Read the model definition and answer for the solid it produces. Units are mm, in the model's axes. A direction names the side the tool comes from. Give positions to 0.01 mm unless a question says otherwise; leave off trailing zeros. Order: outer loops, then holes, each group sorted by start corner. A loop starts at its lowest first (then second) coordinate and runs counter-clockwise, first axis right, second up. Notation, with made-up numbers: (-33, 27.5) - (-29, 27.5) arc R11 cw to (-29, 48.5) - close; hole circle Ø3 at (79.25, -7.5). An arc over 180 degrees is marked (long way). Write item = value, one per line.
```python
from build123d import *

# Parameters (mm, degrees)
SKETCH1_W           = 50
SKETCH1_H           = 50
BOSS_EXTRUDE1_DEPTH = 2
SKETCH2_W           = 50
SKETCH2_H           = 50
SKETCH2_W_2         = 38
SKETCH2_H_2         = 38
BOSS_EXTRUDE2_DEPTH = 23


with BuildPart() as part:
    # Sketch1 → Boss-Extrude1 (new body)
    with BuildSketch(Plane.XY):
        Rectangle(SKETCH1_W, SKETCH1_H)
        with BuildLine():
            Line((12.263455967, 16.763455967), (-12.263455967, 16.763455967))
            ThreePointArc((-12.263455967, 16.763455967), (-15.445436483, 15.445436483), (-16.763455967, 12.263455967))
            Line((-16.763455967, 12.263455967), (-16.763455967, -12.263455967))
            ThreePointArc((-16.763455967, -12.263455967), (-15.445436483, -15.445436483), (-12.263455967, -16.763455967))
            Line((-12.263455967, -16.763455967), (12.263455967, -16.763455967))
            ThreePointArc((12.263455967, -16.763455967), (15.445436483, -15.445436483), (16.763455967, -12.263455967))
            Line((16.763455967, -12.263455967), (16.763455967, 12.263455967))
            ThreePointArc((16.763455967, 12.263455967), (15.445436483, 15.445436483), (12.263455967, 16.763455967))
        make_face(mode=Mode.SUBTRACT)
    extrude(amount=-BOSS_EXTRUDE1_DEPTH)

    # Sketch2 → Boss-Extrude2 (add)
    with BuildSketch(Plane(origin=(0, 0, -2), x_dir=(-1, 0, 0), z_dir=(0, 0, -1))):
        Rectangle(SKETCH2_W, SKETCH2_H)
        Rectangle(SKETCH2_W_2, SKETCH2_H_2, mode=Mode.SUBTRACT)
    extrude(amount=BOSS_EXTRUDE2_DEPTH)


solid = part.part
```
1. Section D-D (y = -18) is taken. Determine the outline of the cut face in (x, z), and give its area (3 significant figures).
Recorded:
outline = (-25, -25) - (-19, -25) - (-19, -2) - (19, -2) - (19, -25) - (25, -25) - (25, 0) - (-25, 0) - close
area = 376 mm^2
2. Straight lines are drawn through the part: L1, parallel to Y at x = 12.5, z = -10.5; L2, parallel to Z at x = 18.5, y = -4. For each, find the intervals that lie inside material, in ascending order. Write a range as [from, to].
Recorded:
L1 = [-25, -19], [19, 25]
L2 = [-2, 0]
3. Flat-ended cylindrical pins translate along their axes: pin 1 (6 mm diameter, centred on x = -7.5, y = -11, fed in from -Z); pin 2 (1.5 mm diameter, centred on x = 11, y = -18.5, fed in from -Z). Find the tip coordinate at first contact, or state that the pin passes through.
Recorded:
pin_1 = through
pin_2 = -25
4. Determine the mould class of faces 1 (the face through (-25, 0, -12)), 2 (the face through (0, 25, -12)), 3 (the face through (15.48, 15.41, -0.99)), 4 (the face through (0, 16.763, -1)) for opening direction X: +X half, -X half, draft (parallel to the pull), parting line (faces both ways), or undercut.
Recorded:
face_1 = -X half
face_2 = draft
face_3 = undercut
face_4 = undercut
5. Section A-A (z = -9.75) is taken. Determine the outline of the cut face in (x, y).
Recorded:
outline = (-25, -25) - (25, -25) - (25, 25) - (-25, 25) - close; hole (-19, -19) - (19, -19) - (19, 19) - (-19, 19) - close
6. Section B-B (x = -8) is taken. Determine the outline of the cut face in (y, z).
Recorded:
outline = (-25, -25) - (-19, -25) - (-19, -2) - (-16.76, -2) - (-16.76, 0) - (-25, 0) - close; (16.76, -2) - (19, -2) - (19, -25) - (25, -25) - (25, 0) - (16.76, 0) - close
7. For faces 5 (the face through (-16.763, 0, -1)), 6 (the face through (19, 0, -13)), 7 (the face through (0, -25, -12)), determine the directions among +Z, -Z, +X, -X, +Y, -Y from which every point of the face is accessible in a straight line to the end or side of a thin tool.
Recorded:
face_5 = +Z, -Z
face_6 = -Z
face_7 = +Z, -Z, +X, -X, -Y
